Geometry: see drawing. Coordinates: mm, zero at the bounding-box minimum. A direction names the side the tool comes from. Give positions to 0.01 mm unless a question says otherwise; leave off trailing zeros. Loops run counter-clockwise (first coordinate to the right, second up) from the corner with the lowest first, then second, coordinate; pieces in that order, holes last. Notation, with made-up numbers: M 83,71 L 128,71 A12 ccw 128,86 Z; hole C 3,12 d6. An arc over 180 degrees is marked long. Answer in a Markdown table with one row per item.
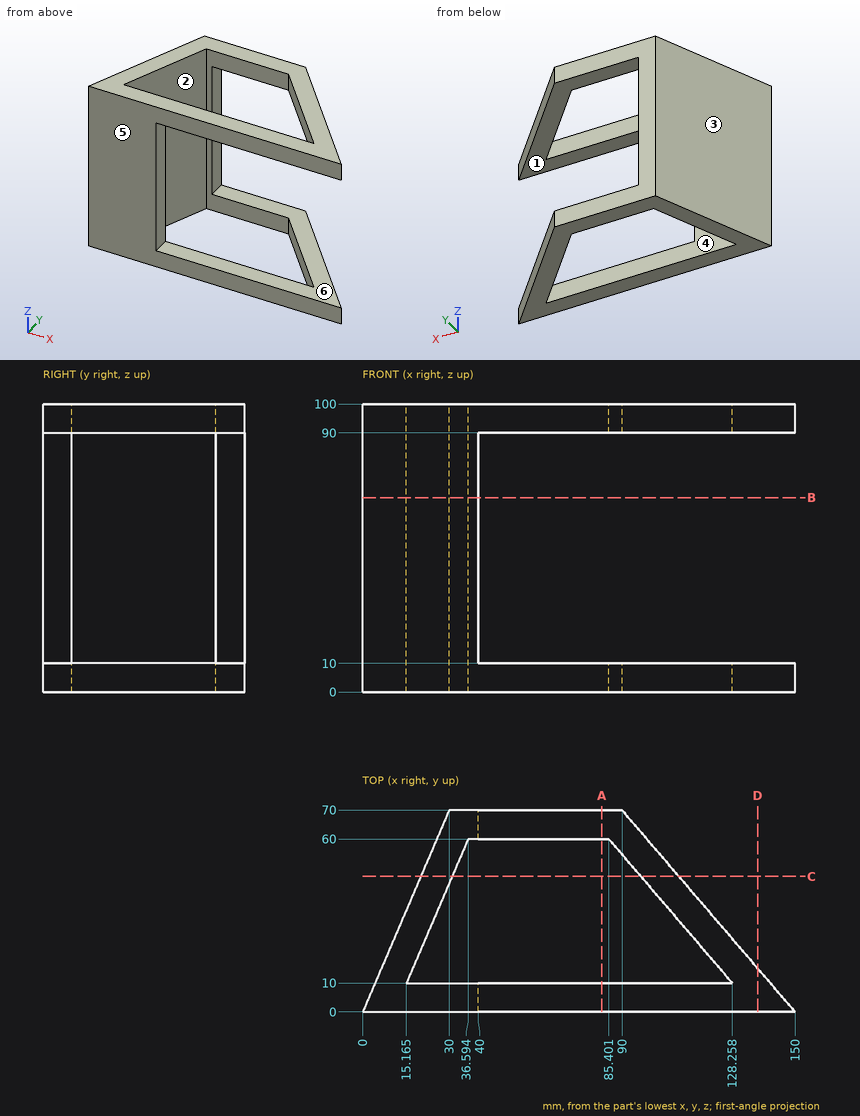
1) Section C-C, the plane y = 47. Return loops of the section in (x, z) (1 decimal), then the cut area to 3 significant figures.
Reply:
| item | result |
|---|---|
| outline | M 20.1,0 L 31,0 L 31,100 L 20.1,100 Z; M 96.5,0 L 109.7,0 L 109.7,10 L 96.5,10 Z; M 96.5,90 L 109.7,90 L 109.7,100 L 96.5,100 Z |
| area | 1,350 mm² |
2) Set-up query: the marked faces 5 and 6. Return all of +Z, -Z, +X, -X, +Y, -Y with unobstructed straight access to the full face (end or side cutting, diameter ignored); none if empty.
Reply:
| item | result |
|---|---|
| face 5 | +Z, -Z, +X, -X, -Y |
| face 6 | +X, +Y, -Y |
3) Pull-direction query (Y, two-part tool) for the marked faces 1, 2, 3 and 4; classes: released by +Y, released by -Y, zero draft, split by the parting line, or undercut.
Reply:
| item | result |
|---|---|
| face 1 | zero draft |
| face 2 | undercut |
| face 3 | released by +Y |
| face 4 | undercut |
4) Section B-B, the plane z = 67.5. Return loops of the section in (x, y) (1 decimal).
Reply:
| item | result |
|---|---|
| outline | M 0,0 L 40,0 L 40,10 L 15.2,10 L 36.6,60 L 40,60 L 40,70 L 30,70 Z |
5) Pin query (flat end, axial travel): pin 1 Ø2 at (y, z) = (51, 40) entering from +X (1 decimal); pin 2 Ø10 at (y, z) = (50, 70) entering from -X (1 decimal); pin 3 Ø5 at (y, z) = (2.5, 41) entering from +X. Return the tip coordinate at first contact, or that it passes through.
Reply:
| item | result |
|---|---|
| pin 1 | stops at x = 33.2 |
| pin 2 | stops at x = 19.3 |
| pin 3 | stops at x = 40 |
6) Material intervals for L1, parallel to Y at x = 46.5, z = 91.5; L2, parallel to X at y = 28.5, z = 6.5 (1 decimal); L3, parallel to X at y = 66, z = 20.5 (1 decimal), sorted ascending.
Reply:
| item | result |
|---|---|
| L1 | y = 0 to 10, 60 to 70 |
| L2 | x = 12.2 to 23.1, 112.4 to 125.6 |
| L3 | x = 28.3 to 40 |
7) Section D-D, the plane x = 137. Return loops of the section in (y, z), then the cut area to 3 significant figures.
Reply:
| item | result |
|---|---|
| outline | M 0,0 L 15.17,0 L 15.17,10 L 0,10 Z; M 0,90 L 15.17,90 L 15.17,100 L 0,100 Z |
| area | 303 mm² |
8) Section A-A, the plane x = 83. Return loops of the section in (y, z), then the cut area to 3 significant figures.
Reply:
| item | result |
|---|---|
| outline | M 0,0 L 10,0 L 10,10 L 0,10 Z; M 0,90 L 10,90 L 10,100 L 0,100 Z; M 60,0 L 70,0 L 70,10 L 60,10 Z; M 60,90 L 70,90 L 70,100 L 60,100 Z |
| area | 400 mm² |
